Can you work these out from the model? Positions are in its coordinate system, mm. Face numbers are marked on the shaded views. A direction names the side the tool comes from. Round coordinates to 2 decimals unless told otherwise and drop trailing zeros. Loops run counter-clockwise (first coordinate to the right, second up) from the corner with the lowest first, then second, coordinate; pieces in that order, holes last. Notation, with made-up numbers: M 63.5,4 L 68.5,4 A31 cw 68.5,30 Z; hole C 12,-13 d4. An arc over 180 degrees is marked long. Answer as CSV lines item,"result".
from build123d import *

# Parameters (mm, degrees)
SKETCH1_W           = 20
SKETCH1_H           = 30
BOSS_EXTRUDE1_DEPTH = 3
SKETCH3_W           = 7
SKETCH3_H           = 14
BOSS_EXTRUDE2_DEPTH = 3
SKETCH4_W           = 3
SKETCH4_H           = 14
BOSS_EXTRUDE3_DEPTH = 15
FILLET1_R           = 1
FILLET2_R           = 1


with BuildPart() as part:
    # Sketch1 → Boss-Extrude1 (new body)
    with BuildSketch(Plane.XY):
        with Locations((10, -15)):
            Rectangle(SKETCH1_W, SKETCH1_H)
    extrude(amount=BOSS_EXTRUDE1_DEPTH)

    # Sketch3 → Boss-Extrude2 (add)
    with BuildSketch(Plane.ZY.offset(-20)):
        with Locations((6.5, -15)):
            Rectangle(SKETCH3_W, SKETCH3_H)
    extrude(amount=BOSS_EXTRUDE2_DEPTH)

    # Sketch4 → Boss-Extrude3 (add)
    with BuildSketch(Plane.ZY.offset(-17)):
        with Locations((8.5, -15)):
            Rectangle(SKETCH4_W, SKETCH4_H)
    extrude(amount=-BOSS_EXTRUDE3_DEPTH)

    # Fillet1
    fillet1_edges = [part.edges().sort_by_distance(p)[0] for p in [
        (20, -4, 3),
        (18.5, -8, 3),
        (20, -22, 5),
        (18.5, -22, 3),
        (24.5, -22, 10),
        (24.5, -8, 10),
        (17, -15, 3),
        (17, -22, 6.5),
        (17, -15, 10),
        (17, -8, 6.5),
        (20, -8, 5),
        (32, -15, 10),
        (32, -22, 8.5),
        (32, -15, 7),
        (26, -22, 7),
        (32, -8, 8.5),
        (26, -8, 7),
        (20, -15, 7),
        (20, -26, 3),
    ]]
    fillet(fillet1_edges, radius=FILLET1_R)

    # Fillet2
    fillet2_edges = [part.edges().sort_by_distance(p)[0] for p in [
        (0, -15, 3),
        (9.5, 0, 3),
        (9.5, -30, 3),
        (0, -15, 0),
        (20, -30, 1),
        (20, 0, 1),
        (10, 0, 0),
        (19.707106781, -30, 2.707106781),
        (19.707106781, 0, 2.707106781),
        (20, -15, 0),
        (10, -30, 0),
        (0, -30, 1.5),
        (0, 0, 1.5),
    ]]
    fillet(fillet2_edges, radius=FILLET2_R)


solid = part.part
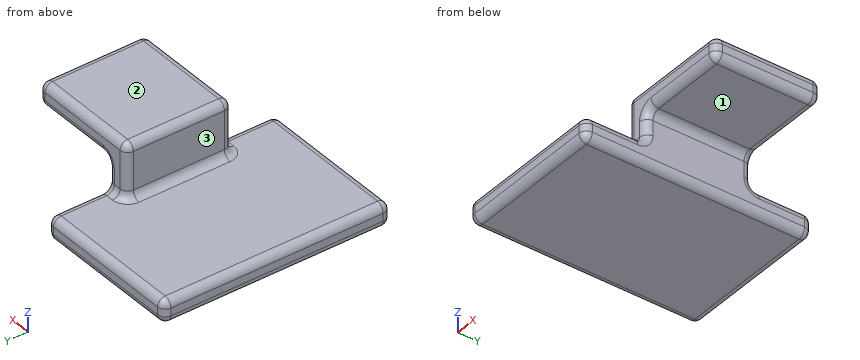
Item 1: If we section it at B-B on z = 5.25: Write out the boundary of the cut face in (x, y).
Output:
outline,"M 17,-21 A1 ccw 18,-22 L 19,-22 A1 ccw 20,-21 L 20,-9 A1 ccw 19,-8 L 18,-8 A1 ccw 17,-9 Z"
Item 2: If we section it at A-A on x = 23: Write out the boundary of the cut face in (y, z), then the cut area to 3 significant figures.
Output:
outline,"M -22,8 A1 ccw -21,7 L -9,7 A1 ccw -8,8 L -8,9 A1 ccw -9,10 L -21,10 A1 ccw -22,9 Z"
area,"41.1 mm2"
Item 3: If we section it at C-C on y = -14.5: Write out the boundary of the cut face in (x, z), then the cut area to 3 significant figures.
Output:
outline,"M 0,1 A1 ccw 1,0 L 19,0 A1 ccw 20,1 L 20,6 A1 cw 21,7 L 31,7 A1 ccw 32,8 L 32,9 A1 ccw 31,10 L 18,10 A1 ccw 17,9 L 17,4 A1 cw 16,3 L 1,3 A1 ccw 0,2 Z"
area,"116 mm2"
Item 4: Will these pins go through, and if not, where does the flat tip stop? pin 1 (1 mm diameter, centred on y = -16.5, z = 6, fed in from -X); pin 2 (5.5 mm diameter, centred on x = 23.5, z = 7.5, fed in from +Y); pin 3 (6 mm diameter, centred on x = 28, y = -18, fed in from -Z).
Output:
pin 1,"stops at x = 17"
pin 2,"stops at y = -8"
pin 3,"stops at z = 7"
Item 5: On a 3-axis mill with a long thin cutter (end or side, diameter ignored), from which of +Z, -Z, +X, -X, +Y, -Y can I reach the whole of each face in a straight line? I mean the marked faces 1, 2 and 3. Say none if no direction works.
Output:
face 1,"-Z, +X, +Y, -Y"
face 2,"+Z, +X, -X, +Y, -Y"
face 3,"+Z, -X, +Y, -Y"
Item 6: If I drill on line 1 along X through (y, z) = (-23, 1.5); line 2 along X through (y, z) = (-18.75, 5.75); line 3 along Z through (x, y) = (10, -4.75), over which ranges is the centre line in solid material (lowest first)? Write a range as from..to.
Output:
line 1,"x = 0..20"
line 2,"x = 17..20"
line 3,"z = 0..3"
